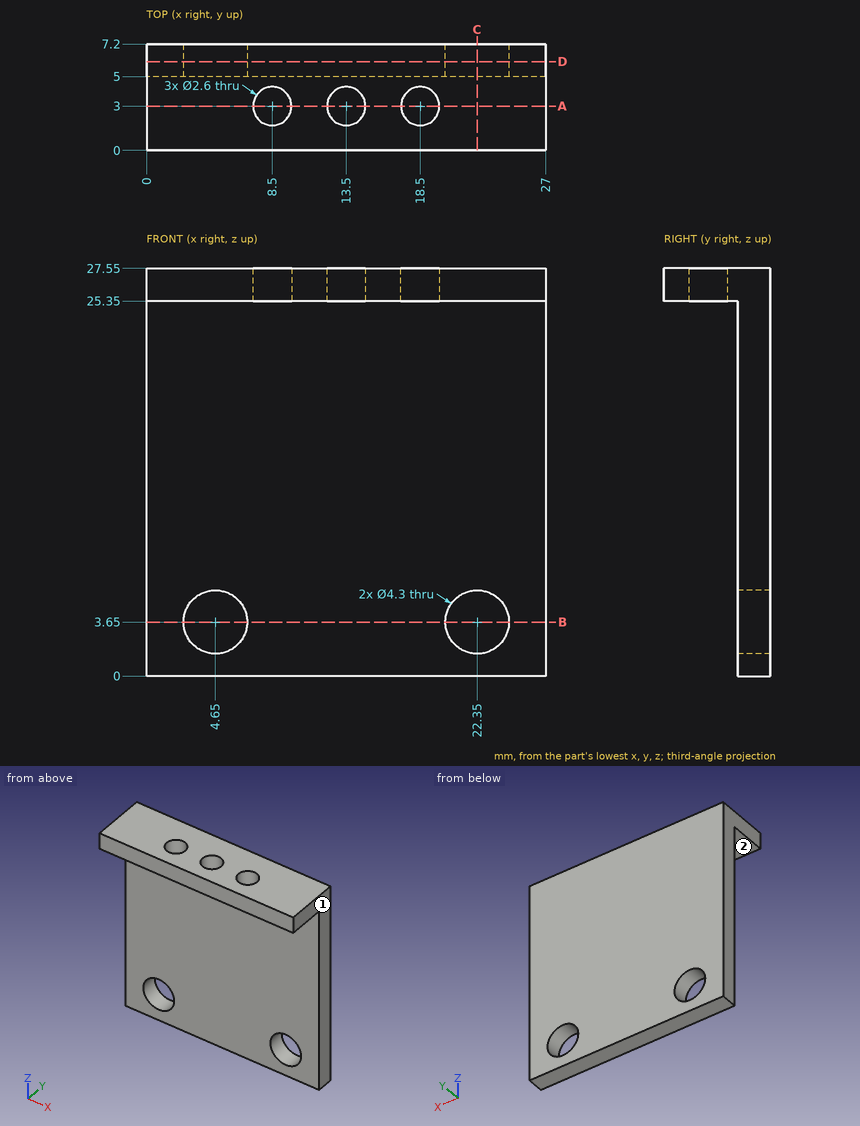
For this review, use the dimensioned drawing (mm, ordinates from the lowest corner) and the shaded views. A direction names the side the tool comes from. Give positions to 0.01 mm unless a question says otherwise; leave off trailing zeros. Write each loop counter-clockwise with the first axis right and the second up, starting at its lowest first coordinate (ties: lowest second). Pieces come first, ordered by that corner, then holes. Notation, with made-up numbers: M 14.5,38 L 22.5,38 A18 ccw 22.5,49 Z; hole C 7.25,7.25 d5. An arc over 180 degrees is marked long. Answer as a JSON object with one key per item and string values. Group by question number.
Item 1: Consider section D-D on y = 6. Write out the cut boundary in (x, z).
Item 2: Consider section C-C on x = 22.35. Write out the cut boundary in (y, z), plus the area to 4 significant figures.
Item 3: Tool access review of the marked faces 1 and 2: name each direction out of +Z, -Z, +X, -X, +Y, -Y from which nothing blocks a thin tool from reaching the whole face with its end or side.
Item 4: Consider section A-A on y = 3. Write out the cut boundary in (x, z).
Item 5: Consider section B-B on z = 3.65. Write out the cut boundary in (x, y).
Item 6: For pin 1 Ø5 at (x, z) = (23.5, 8.5) entering from -Y; pin 2 Ø1.5 at (x, y) = (13, 1.5) entering from -Z, all flat-tipped, find the tip position at first contact; note any pin that passes through.
Item 7: For probe 1 along Y at (x, z) = (8.5, 26.8); probe 2 along Z at (x, y) = (4.65, 5.6); probe 3 along Z at (x, y) = (19.75, 4), list the stretches that pass through material, from the lowest coordinate up. Write a range as [from, to].
Check result:
{
 "1": {"outline": "M 0,0 L 27,0 L 27,27.55 L 0,27.55 Z; hole C 4.65,3.65 d4.3; hole C 22.35,3.65 d4.3"},
 "2": {"outline": "M 0,25.35 L 5,25.35 L 5,5.8 L 7.2,5.8 L 7.2,27.55 L 0,27.55 Z; M 5,0 L 7.2,0 L 7.2,1.5 L 5,1.5 Z", "area": "62.15 mm^2"},
 "3": {"face 1": "+Z, -Z, +X, +Y, -Y", "face 2": "-Z, +X, -X, -Y"},
 "4": {"outline": "M 0,25.35 L 7.2,25.35 L 7.2,27.55 L 0,27.55 Z; M 9.8,25.35 L 12.2,25.35 L 12.2,27.55 L 9.8,27.55 Z; M 14.8,25.35 L 17.2,25.35 L 17.2,27.55 L 14.8,27.55 Z; M 19.8,25.35 L 27,25.35 L 27,27.55 L 19.8,27.55 Z"},
 "5": {"outline": "M 0,5 L 2.5,5 L 2.5,7.2 L 0,7.2 Z; M 6.8,5 L 20.2,5 L 20.2,7.2 L 6.8,7.2 Z; M 24.5,5 L 27,5 L 27,7.2 L 24.5,7.2 Z"},
 "6": {"pin 1": "stops at y = 5", "pin 2": "stops at z = 25.35"},
 "7": {"probe 1": "y = [0, 1.7], [4.3, 7.2]", "probe 2": "z = [0, 1.5], [5.8, 27.55]", "probe 3": "z = [25.35, 27.55]"}
}
